Check sheet for the drawn part. Datum: minimum x, y, z corner. Units: mm. A direction names the side the tool comes from. Give positions to 0.01 mm unless a question says otherwise; leave off trailing zeros. Order: outer loops, then holes, each group sorted by start corner. A loop starts at its lowest first (then second) coordinate and runs counter-clockwise, first axis right, second up. Notation, with made-up numbers: (53, 5.25) - (93, 5.25) arc R20 ccw to (93, 18.25) - close; hole circle Ø3 at (49.25, 57). An arc over 180 degrees is marked (long way). Answer as a JSON object with one key per item and string values. Group by question number.
(1) Depth check by flat-ended pin: pin 1 Ø2.5 at (x, z) = (53.5, 11.5) entering from +Y; pin 2 Ø8 at (x, z) = (27.75, 10.5) entering from -Y. Enter the tip coordinate at first touch or a pass-through.
(2) Section check B-B (y = 6). Record the boundary of the cut face in (x, z).
(3) Thickness scan on line 1 (Y direction, x = 43, z = 10.5); line 2 (Y direction, x = 14, z = 3.75); line 3 (Z direction, x = 27.75, y = 31). Record the ranges inside material, lowest first.
(4) Mould release check, pull along Y, two halves, no side actions. Record for the marked faces 5, 6 and 7: +Y half, -Y half, draft (parallel to the pull), parting line (faces both ways), or undercut.
(5) Access from +Z, -Z, +X, -X, +Y, -Y to the whole of each face (thin tool, end or side, straight path). Record for the marked faces 1, 2, 3 and 4.
(6) Section check A-A (x = 47). Record the boundary of the cut face in (y, z).
(7) Section check D-D (y = 71). Record the boundary of the cut face in (x, z), then the cut area to 4 significant figures.
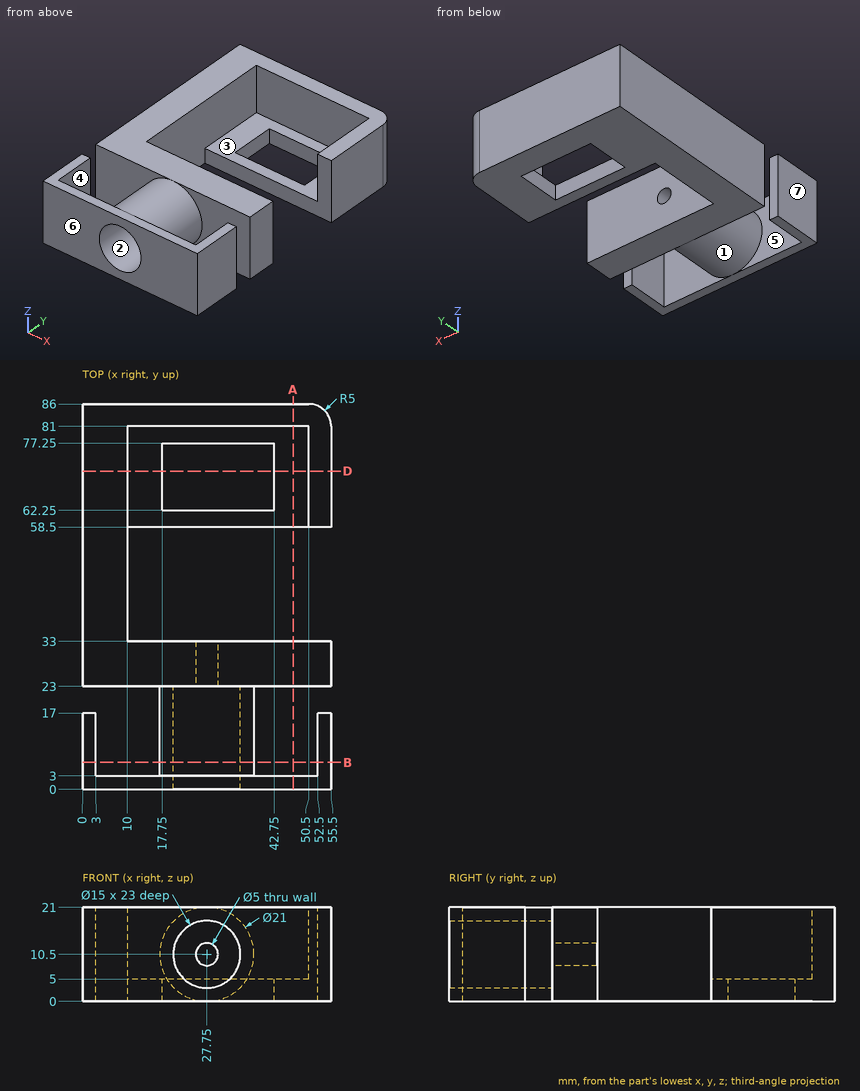
Solutions:
{
 "1": {"pin 1": "stops at y = 85.68", "pin 2": "stops at y = 23"},
 "2": {"outline": "(0, 0) - (3, 0) - (3, 21) - (0, 21) - close; circle Ø21 at (27.75, 10.5); (52.5, 0) - (55.5, 0) - (55.5, 21) - (52.5, 21) - close; hole circle Ø15 at (27.75, 10.5)"},
 "3": {"line 1": "y = 0 to 3, 23 to 33, 81 to 86", "line 2": "y = 0 to 3, 23 to 33, 58.5 to 86", "line 3": "z = 0 to 8, 13 to 21"},
 "4": {"face 5": "undercut", "face 6": "-Y half", "face 7": "draft"},
 "5": {"face 1": "none", "face 2": "-Y", "face 3": "+Z", "face 4": "+Z, -Z"},
 "6": {"outline": "(0, 0) - (3, 0) - (3, 21) - (0, 21) - close; (23, 0) - (33, 0) - (33, 21) - (23, 21) - close; (58.5, 0) - (86, 0) - (86, 21) - (81, 21) - (81, 5) - (58.5, 5) - close"},
 "7": {"outline": "(0, 0) - (17.75, 0) - (17.75, 5) - (10, 5) - (10, 21) - (0, 21) - close; (42.75, 0) - (55.5, 0) - (55.5, 21) - (50.5, 21) - (50.5, 5) - (42.75, 5) - close", "area": "392.5 mm2"}
}
